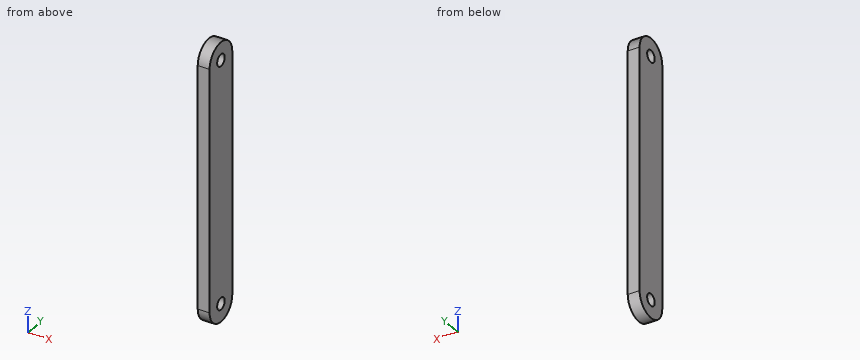
```python
from build123d import *

# Parameters (mm, degrees)
SKETCH1_R           = 2.4
BOSS_EXTRUDE1_DEPTH = 5
SCALE1_SCALE        = 0.8
SKETCH2_R           = 2
CUT_EXTRUDE1_DEPTH  = 47.561786907
SKETCH4_R           = 2
BOSS_EXTRUDE2_DEPTH = 4
BOSS_EXTRUDE3_DEPTH = 4
SKETCH7_R           = 2
CUT_EXTRUDE2_DEPTH  = 48.334629336


with BuildPart() as part:
    # Sketch1 → Boss-Extrude1 (new body)
    with BuildSketch(Plane(origin=(0, 0, 0), x_dir=(0, 0, -1), z_dir=(1, 0, 0))):
        with BuildLine():
            Line((-50, 7.5), (50, 7.5))
            ThreePointArc((50, 7.5), (57.5, 0), (50, -7.5))
            Line((50, -7.5), (-50, -7.5))
            ThreePointArc((-50, -7.5), (-57.5, 0), (-50, 7.5))
        make_face()
        with Locations((-50, 0)):
            Circle(SKETCH1_R, mode=Mode.SUBTRACT)
        with Locations((50, 0)):
            Circle(SKETCH1_R, mode=Mode.SUBTRACT)
    extrude(amount=BOSS_EXTRUDE1_DEPTH)


with BuildPart() as part_1:
    # Scale1: scaled about (2.5, 0, 0)
    add(part.part.scale(SCALE1_SCALE).moved(Location((0.5, 0, 0))))

    # Sketch2 → Cut-Extrude1 (cut, through all)
    with BuildSketch(Plane(origin=(4.5, 0, 0), x_dir=(0, 0, -1), z_dir=(1, 0, 0))):
        with Locations((-40, 0)):
            Circle(SKETCH2_R)
        with Locations((40, 0)):
            Circle(SKETCH2_R)
    extrude(amount=-CUT_EXTRUDE1_DEPTH, mode=Mode.SUBTRACT)

    # Sketch4 → Boss-Extrude2 (add, through all)
    with BuildSketch(Plane.ZY.offset(-0.5)):
        with Locations((-40, 0)):
            Circle(SKETCH4_R)
    extrude(amount=-BOSS_EXTRUDE2_DEPTH)

    # Sketch6 → Boss-Extrude3 (add, through all)
    with BuildSketch(Plane.ZY.offset(-0.5)):
        with BuildLine():
            Line((-40.78212409, -6), (-33.634711985, -6))
            Line((-33.634711985, -6), (-33.634711985, 6))
            Line((-33.634711985, 6), (-40.78212409, 6))
            ThreePointArc((-40.78212409, 6), (-46.78212409, 0), (-40.78212409, -6))
        make_face()
    extrude(amount=-BOSS_EXTRUDE3_DEPTH)

    # Sketch7 → Cut-Extrude2 (cut, through all)
    with BuildSketch(Plane.ZY.offset(-0.5)):
        with Locations((-40.78760592, 0)):
            Circle(SKETCH7_R)
    extrude(amount=-CUT_EXTRUDE2_DEPTH, mode=Mode.SUBTRACT)


solid = part_1.part
```
CAD build for the part. Positions are in the model's coordinates, mm. Give positions to 0.01 mm unless a question says otherwise; leave off trailing zeros. Loops run counter-clockwise (first coordinate to the right, second up) from the corner with the lowest first, then second, coordinate; pieces in that order, holes last. Notation, with made-up numbers: (83.25, -11.75) - (125.25, -11.75) arc R13 cw to (125.25, 7.25) - close; hole circle Ø9 at (-19, 46). An arc over 180 degrees is marked (long way). Put each result on its own line as item: value.
Q1. Slice it at B-B (x = 2.2). Give the cut face in (y, z), plus the area to 3 significant figures.
Filled in:
outline: (-6, -40.78) arc R6 ccw to (6, -40.78) - (6, 40) arc R6 ccw to (-6, 40) - close; hole circle Ø4 at (0, -40.79); hole circle Ø4 at (0, 40)
area: 1,060 mm²
Q2. Slice it at A-A (y = 0). Give the cut face in (x, z), plus the area to 3 significant figures.
Filled in:
outline: (0.5, -46.78) - (4.5, -46.78) - (4.5, -42.79) - (0.5, -42.79) - close; (0.5, -38.79) - (4.5, -38.79) - (4.5, 38) - (0.5, 38) - close; (0.5, 42) - (4.5, 42) - (4.5, 46) - (0.5, 46) - close
area: 339 mm²
Q3. Slice it at C-C (y = -4.5). Give the cut face in (x, z).
Filled in:
outline: (0.5, -44.75) - (4.5, -44.75) - (4.5, 43.97) - (0.5, 43.97) - close
Q4. Probe line 1 along Z through (x, y) = (4, -0.25); line 2 along Y through (x, z) = (2.25, 40); line 3 along Z through (x, y) = (1.95, 1.25). List the from-to ranges inside material, lowest first.
Filled in:
line 1: z = -46.78 to -42.77, -38.8 to 38.02, 41.98 to 45.99
line 2: y = -6 to -2, 2 to 6
line 3: z = -46.65 to -42.35, -39.23 to 38.44, 41.56 to 45.87
Q5. Flat gauge pins, fed straight in: pin 1 (1 mm diameter, centred on x = 3.5, y = -4, fed in from -Z); pin 2 (1 mm diameter, centred on x = 1.5, y = -2.5, fed in from -Z). Where does each tip first touch, or does it go through?
Filled in:
pin 1: stops at z = -45.66
pin 2: stops at z = -46.44
